For this review, take the finished solid that the model builds, in its own axes (mm). A direction names the side the tool comes from. Give positions to 0.01 mm unless a question says otherwise; leave off trailing zeros. Order: outer loops, then holes, each group sorted by start corner. A loop starts at its lowest first (then second) coordinate and runs counter-clockwise, first axis right, second up.
from build123d import *

# Parameters (mm, degrees)
SKETCH1_W                = 120
SKETCH1_H                = 49
BOSS_EXTRUDE1_DEPTH      = 12.5
SKETCH2_W                = 95
SKETCH2_H                = 39
CUT_EXTRUDE1_DEPTH       = 20
FILLET1_R                = 2
M3_START                 = -60
M3_CLEARANCE_SLOT1_DEPTH = 3
SKETCH6_R                = 5.5
CUT_EXTRUDE2_DEPTH       = 20
SKETCH7_R                = 1.5
CUT_EXTRUDE3_DEPTH       = 79.468146403


# Read off the part's stored shape, not the designer's step: M3 Clearance Slot1
with BuildPart() as part:
    # Sketch1 → Boss-Extrude1 (new, symmetric)
    with BuildSketch(Plane(origin=(0, 0, 0), x_dir=(1, 0, 0), z_dir=(0, 1, 0))):
        Rectangle(SKETCH1_W, SKETCH1_H)
    extrude(amount=BOSS_EXTRUDE1_DEPTH, both=True)

    # Sketch2 → Cut-Extrude1 (cut)
    with BuildSketch(Plane(origin=(0, 12.5, 0), x_dir=(1, 0, 0), z_dir=(0, 1, 0))):
        with Locations((-9.5, 0)):
            Rectangle(SKETCH2_W, SKETCH2_H)
    extrude(amount=-CUT_EXTRUDE1_DEPTH, mode=Mode.SUBTRACT)

    # Fillet1
    fillet1_edges = [part.edges().sort_by_distance(p)[0] for p in [
        (0, 12.5, 24.5),
        (60, 12.5, 0),
        (0, 12.5, -24.5),
    ]]
    fillet(fillet1_edges, radius=FILLET1_R)

    # M3 Clearance Slot1 outline → M3 Clearance Slot1 (cut)
    with BuildSketch(Plane.YZ.offset(M3_START)):
        with BuildLine():
            Line((4.2, -14), (4.2, -11))
            ThreePointArc((4.2, -11), (2.5, -9.3), (0.8, -11))
            Line((0.8, -11), (0.8, -14))
            ThreePointArc((0.8, -14), (2.5, -15.7), (4.2, -14))
        make_face()
        with BuildLine():
            ThreePointArc((4.2, 14), (2.5, 15.7), (0.8, 14))
            Line((0.8, 14), (0.8, 11))
            ThreePointArc((0.8, 11), (2.5, 9.3), (4.2, 11))
            Line((4.2, 11), (4.2, 14))
        make_face()
    extrude(amount=M3_CLEARANCE_SLOT1_DEPTH, mode=Mode.SUBTRACT)

    # Sketch6 → Cut-Extrude2 (cut)
    with BuildSketch(Plane.XZ.offset(12.5)):
        with Locations(Location((48, 0, 0), (0, 0, 270))):
            Circle(SKETCH6_R)
    extrude(amount=-CUT_EXTRUDE2_DEPTH, mode=Mode.SUBTRACT)

    # Sketch7 → Cut-Extrude3 (cut, through all)
    with BuildSketch(Plane(origin=(0, 0, -24.5), x_dir=(-1, 0, 0), z_dir=(0, 0, -1))):
        with Locations((-48, 1.5)):
            Circle(SKETCH7_R)
    extrude(amount=-CUT_EXTRUDE3_DEPTH, mode=Mode.SUBTRACT)


solid = part.part
1) Draft analysis for pull direction X (two halves, no side actions). For faces 1 (the face through (-58.5, 2.5, 9.3)), 2 (the face through (49.652, -2.64, -5.246)), 3 (the face through (60, -1, 0)), 4 (the face through (48, 7.5, 0)), state which applies: +X half, -X half, draft (parallel to the pull), parting line (faces both ways), or undercut.
Answer sheet:
face 1: draft
face 2: undercut
face 3: +X half
face 4: undercut
2) Clearance check with flat-ended pins moving along their axes: pin 1 (1.8 mm diameter, centred on x = 48, y = 1.5, fed in from +Z); pin 2 (12 mm diameter, centred on x = 3.5, z = -3, fed in from +Y); pin 3 (12 mm diameter, centred on x = 50, z = -2, fed in from -Y). State where each tip first meets the part, or that it passes through.
Answer sheet:
pin 1: passes through
pin 2: stops at y = -7.5
pin 3: stops at y = -12.5
3) To check wall thickness, follow line 1 (X direction, y = 1.5, z = 15.5); line 2 (X direction, y = 1.5, z = 13.25); line 3 (Y direction, x = 48, z = -11). State the ranges of each line that lie inside material, in increasing order.
Answer sheet:
line 1: x = -60 to -57, 38 to 46.5, 49.5 to 60
line 2: x = 38 to 46.5, 49.5 to 60
line 3: y = -12.5 to 0, 3 to 12.5
4) We need section C-C on x = 0.5. Give the boundary of the cut face in (y, z), then the cut area to 3 significant figures.
Answer sheet:
outline: (-12.5, -24.5) - (10.5, -24.5) arc R2 ccw to (12.5, -22.5) - (12.5, -19.5) - (-7.5, -19.5) - (-7.5, 19.5) - (12.5, 19.5) - (12.5, 22.5) arc R2 ccw to (10.5, 24.5) - (-12.5, 24.5) - close
area: 443 mm2
5) We need section B-B on z = 7.5. Give the boundary of the cut face in (x, y), then the cut area to 3 significant figures.
Answer sheet:
outline: (-60, -12.5) - (60, -12.5) - (60, 10.5) arc R2 ccw to (58, 12.5) - (38, 12.5) - (38, -7.5) - (-57, -7.5) - (-57, 12.5) - (-60, 12.5) - close; hole circle Ø3 at (48, 1.5)
area: 1,090 mm2
6) We need section A-A on y = -5. Give the boundary of the cut face in (x, z), then the cut area to 3 significant figures.
Answer sheet:
outline: (-60, -24.5) - (60, -24.5) - (60, 24.5) - (-60, 24.5) - close; hole (-57, -19.5) - (38, -19.5) - (38, 19.5) - (-57, 19.5) - close; hole circle Ø11 at (48, 0)
area: 2,080 mm2
7) We need section D-D on z = 0. Give the boundary of the cut face in (x, y), then the cut area to 3 significant figures.
Answer sheet:
outline: (-60, -12.5) - (42.5, -12.5) - (42.5, 7.5) - (53.5, 7.5) - (53.5, -12.5) - (60, -12.5) - (60, 10.5) arc R2 ccw to (58, 12.5) - (38, 12.5) - (38, -7.5) - (-57, -7.5) - (-57, 12.5) - (-60, 12.5) - close
area: 879 mm2
8) Tool access review of faces 5 (the face through (-59, 4.2, 12)), 6 (the face through (59.4, 11.93, -0.34)), 7 (the face through (-10, 3, 19.5)): name each direction out of +Z, -Z, +X, -X, +Y, -Y from which nothing blocks a thin tool from reaching the whole face with its end or side.
Answer sheet:
face 5: -X
face 6: +Z, -Z, +X, +Y
face 7: +Y
